Here's how the part is built. I have some questions about the finished solid (model axes, mm). Face numbers are marked on the shaded views. A direction names the side the tool comes from. Give positions to 0.01 mm unless a question says otherwise; leave off trailing zeros. Write each loop counter-clockwise with the first axis right and the second up, starting at its lowest first coordinate (ties: lowest second). Pieces come first, ordered by that corner, then holes. Notation, with made-up numbers: (23, 40) - (42, 40) arc R22 cw to (42, 60) - close; hole circle Ø1 at (26.25, 19). An arc over 180 degrees is marked (long way). Write each question's results on one line, items separated by ' | '. Start each with the question number.
Item 1: Suppose I cut it at C-C on z = 21.25. List the corners of the cut face in (x, y) for me.
Item 2: We'd pull the mould along Z, two halves only. Please class the marked faces 1, 2 and 3: +Z half, -Z half, draft (parallel to the pull), parting line (faces both ways), or undercut.
Item 3: Which directions (+Z, -Z, +X, -X, +Y, -Y) give clear straight access to the entire face, cutting with the end or side of a thin tool? Please do the marked faces 4, 5, 6 and 7.
Item 4: Will these pins go through, and if not, where does the flat tip stop? P1, Ø3, axis at y = 6.5, z = 17.5, coming from the -X side; P2, Ø4, axis at x = -4, y = 7.5, coming from the +Z side; P3, Ø2, axis at y = 9.5, z = 22.5, coming from the +X side.
Item 5: Please list where these lines run through material, in increasing order: line 1 along Z through (x, y) = (-1.75, 3.25); line 2 along X through (y, z) = (2.25, 20); line 3 along X through (y, z) = (2, 16.75).
Item 6: Suppose I cut it at D-D on x = -8. List the corners of the cut face in (y, z) for me, then the cut area to 3 significant figures.
Item 7: Suppose I cut it at A-A on x = -2.5. List the corners of the cut face in (y, z) for me.
Item 8: Suppose I cut it at B-B on y = 10.25. Count the separate pieces of the cut face and the enclosed holes in it, then the cut area to 3 significant figures.
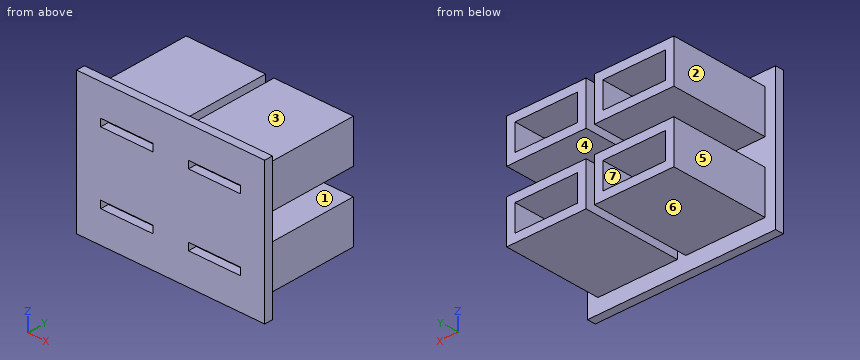
```python
from build123d import *

# Parameters (mm, degrees)
F0_W     = 25.4
F0_H     = 22.86
F1_DEPTH = 1.016
F2_W     = 6.35
F2_H     = 0.889
F3_DEPTH = 25.4
F4_W     = 9.652
F4_H     = 5.207
F4_W_2   = 7.62
F4_H_2   = 3.175
F5_DEPTH = 12.954
F6_W     = 25.4
F6_H     = 2.794
F6_H_2   = 3.048
F7_DEPTH = 12.955
F8_W     = 2.54
F8_H     = 17.018
F9_DEPTH = 25.4


with BuildPart() as f1:
    # F0 (on Front) → F1 (new body)
    with BuildSketch(Plane.XZ):
        with Locations((-10.134171, 23.561226)):
            Rectangle(F0_W, F0_H)
    extrude(amount=-F1_DEPTH)

    # F2 (on face) → F3 (cut)
    with BuildSketch(Plane.XZ):
        with Locations((-14.198171, 27.688726)):
            Rectangle(F2_W, F2_H)
        with Locations((-3.530171, 27.688726)):
            Rectangle(F2_W, F2_H)
        with Locations((-14.198171, 19.179726)):
            Rectangle(F2_W, F2_H)
        with Locations((-3.530171, 19.179726)):
            Rectangle(F2_W, F2_H)
    extrude(amount=-F3_DEPTH, mode=Mode.SUBTRACT)

    # F4 (on face) → F5 (join)
    with BuildSketch(Plane.XZ):
        with Locations((-14.198171, 27.688726)):
            Rectangle(F4_W, F4_H)
        with Locations((-14.198171, 27.688726)):
            Rectangle(F4_W_2, F4_H_2, mode=Mode.SUBTRACT)
        with Locations((-3.530171, 27.688726)):
            Rectangle(F4_W, F4_H)
        with Locations((-3.530171, 27.688726)):
            Rectangle(F4_W_2, F4_H_2, mode=Mode.SUBTRACT)
        with Locations((-14.198171, 19.306726)):
            Rectangle(F4_W, F4_H)
        with Locations((-14.198171, 19.306726)):
            Rectangle(F4_W_2, F4_H_2, mode=Mode.SUBTRACT)
        with Locations((-3.530171, 19.306726)):
            Rectangle(F4_W, F4_H)
        with Locations((-3.530171, 19.306726)):
            Rectangle(F4_W_2, F4_H_2, mode=Mode.SUBTRACT)
    extrude(amount=-F5_DEPTH)

    # F6 (on face) → F7 (cut, through all)
    with BuildSketch(Plane.XZ):
        with Locations((-10.134171, 13.528226)):
            Rectangle(F6_W, F6_H)
        with Locations((-10.134171, 33.467226)):
            Rectangle(F6_W, F6_H_2)
    extrude(amount=-F7_DEPTH, mode=Mode.SUBTRACT)

    # F8 (on face) → F9 (cut)
    with BuildSketch(Plane.XZ):
        with Locations((-21.564171, 23.434226)):
            Rectangle(F8_W, F8_H)
    extrude(amount=-F9_DEPTH, mode=Mode.SUBTRACT)


solid = f1.part
```
Checked values:
1) outline: (-20.29, 0) - (2.57, 0) - (2.57, 1.02) - (1.3, 1.02) - (1.3, 12.95) - (-8.36, 12.95) - (-8.36, 1.02) - (-9.37, 1.02) - (-9.37, 12.95) - (-19.02, 12.95) - (-19.02, 1.02) - (-20.29, 1.02) - close
2) face 1: undercut | face 2: draft | face 3: +Z half
3) face 4: +X, -X, +Y | face 5: +Z, -Z, -X, +Y | face 6: -Z, +X, -X, +Y | face 7: +Y
4) P1: stops at x = -19.02 | P2: stops at z = 30.29 | P3: stops at x = 1.3
5) line 1: z = 16.7 to 17.72, 20.89 to 21.91, 25.09 to 26.1, 29.28 to 30.29 | line 2: x = -19.02 to -18.01, -10.39 to -9.37, -8.36 to -7.34, 0.28 to 1.3 | line 3: x = -19.02 to -9.37, -8.36 to 1.3
6) outline: (0, 14.93) - (1.02, 14.93) - (1.02, 16.7) - (12.95, 16.7) - (12.95, 21.91) - (1.02, 21.91) - (1.02, 25.09) - (12.95, 25.09) - (12.95, 30.29) - (1.02, 30.29) - (1.02, 31.94) - (0, 31.94) - close | area: 142 mm^2
7) outline: (0, 14.93) - (1.02, 14.93) - (1.02, 16.7) - (12.95, 16.7) - (12.95, 17.72) - (1.02, 17.72) - (1.02, 18.74) - (0, 18.74) - close; (0, 19.62) - (1.02, 19.62) - (1.02, 20.89) - (12.95, 20.89) - (12.95, 21.91) - (1.02, 21.91) - (1.02, 25.09) - (12.95, 25.09) - (12.95, 26.1) - (1.02, 26.1) - (1.02, 27.24) - (0, 27.24) - close; (0, 28.13) - (1.02, 28.13) - (1.02, 29.28) - (12.95, 29.28) - (12.95, 30.29) - (1.02, 30.29) - (1.02, 31.94) - (0, 31.94) - close
8) separate pieces: 4 | enclosed holes: 4 | area: 104 mm^2
